```python
from build123d import *

# Parameters (mm, degrees)
F0_W     = 508
F0_H     = 685.8
F1_DEPTH = 31.75
F3_DEPTH = 31.75


with BuildPart() as f1:
    # F0 (on Top) → F1 (new body)
    with BuildSketch(Plane.XY):
        Rectangle(F0_W, F0_H)
    extrude(amount=F1_DEPTH)

    # F2 (on face) → F3 (cut)
    with BuildSketch(Plane.XY.offset(31.75)):
        with BuildLine():
            ThreePointArc((-6.35, 304.8), (0, 298.45), (6.35, 304.8))
            ThreePointArc((6.35, 304.8), (0, 311.15), (-6.35, 304.8))
        make_face()
        with BuildLine():
            ThreePointArc((-6.35, 50.8), (0, 44.45), (6.35, 50.8))
            ThreePointArc((6.35, 50.8), (0, 57.15), (-6.35, 50.8))
        make_face()
        with BuildLine():
            Line((6.35, 50.8), (6.35, 304.8))
            ThreePointArc((6.35, 304.8), (0, 298.45), (-6.35, 304.8))
            Line((-6.35, 304.8), (-6.35, 50.8))
            ThreePointArc((-6.35, 50.8), (0, 57.15), (6.35, 50.8))
        make_face()
    extrude(amount=-F3_DEPTH, mode=Mode.SUBTRACT)


solid = f1.part
```
CAD build for the part. Positions are in the model's coordinates, mm. A direction names the side the tool comes from. Coordinates: 2 decimals unless noted, no trailing zeros. Write each loop counter-clockwise with the first axis right and the second up, starting at its lowest first coordinate (ties: lowest second). Pieces come first, ordered by that corner, then holes.
(1) Two-plate mould, pull along Y, no slides. Class faces 1 (the face through (-4, -342.9, 16)), 2 (the face through (-6.35, 180, 16)), 3 (the face through (-254, -5, 16)): +Y half, -Y half, draft (parallel to the pull), parting line (faces both ways), or undercut.
(2) Drill centre lines: probe 1 along Y at (x, z) = (0, 11); probe 2 along X at (y, z) = (213, 16). Where is each one in solid material? Low to high.
(3) 3-axis set-ups, long thin cutter, end or side, ignore diameter. For faces 4 (the face through (6.35, 176, 16)), 5 (the face through (-4, 5, 0)): which of +Z, -Z, +X, -X, +Y, -Y reach the whole face in a straight line?
(4) Cut at A-A, the plane y = 131. List the corners of the cut face in (x, z), and give its area (3 significant figures).
Geometry says:
1. face 1: -Y half
1. face 2: undercut
1. face 3: draft
2. probe 1: y = -342.9 to 44.45, 311.15 to 342.9
2. probe 2: x = -254 to -6.35, 6.35 to 254
3. face 4: +Z, -Z
3. face 5: -Z, +X, -X, +Y, -Y
4. outline: (-254, 0) - (-6.35, 0) - (-6.35, 31.75) - (-254, 31.75) - close; (6.35, 0) - (254, 0) - (254, 31.75) - (6.35, 31.75) - close
4. area: 15,700 mm2
